from build123d import *

# Parameters (mm, degrees)
SKETCH1_W           = 66.4
SKETCH1_H           = 66.4
BOSS_EXTRUDE1_DEPTH = 59
SKETCH2_R           = 19.075
SKETCH2_R_2         = 2.75
CUT_EXTRUDE1_DEPTH  = 111.900495941
SKETCH3_W           = 57.4
SKETCH3_H           = 54.5
CUT_EXTRUDE2_DEPTH  = 61.9
CUT_EXTRUDE3_DEPTH  = 111.900495941
SKETCH5_W           = 116.4
SKETCH5_H           = 59
BOSS_EXTRUDE2_DEPTH = 4.5
SKETCH6_R           = 2.2
CUT_EXTRUDE4_DEPTH  = 126.166169551


with BuildPart() as part:
    # Sketch1 → Boss-Extrude1 (new body)
    with BuildSketch(Plane.XY):
        with Locations((33.2, 33.2)):
            Rectangle(SKETCH1_W, SKETCH1_H)
    extrude(amount=BOSS_EXTRUDE1_DEPTH)

    # Sketch2 → Cut-Extrude1 (cut, through all)
    with BuildSketch(Plane.XY.offset(59)):
        with Locations((33.2, 33.2)):
            Circle(SKETCH2_R)
        with Locations((9.63, 56.77)):
            Circle(SKETCH2_R_2)
        with Locations((56.77, 56.77)):
            Circle(SKETCH2_R_2)
        with Locations((56.77, 9.63)):
            Circle(SKETCH2_R_2)
        with Locations((9.63, 9.63)):
            Circle(SKETCH2_R_2)
    extrude(amount=-CUT_EXTRUDE1_DEPTH, mode=Mode.SUBTRACT)

    # Sketch3 → Cut-Extrude2 (cut)
    with BuildSketch(Plane(origin=(0, 66.4, 0), x_dir=(1, 0, 0), z_dir=(0, 1, 0))):
        with Locations((33.2, -27.25)):
            Rectangle(SKETCH3_W, SKETCH3_H)
    extrude(amount=-CUT_EXTRUDE2_DEPTH, mode=Mode.SUBTRACT)

    # Sketch4 → Cut-Extrude3 (cut, through all)
    with BuildSketch(Plane(origin=(66.4, 0, 0), x_dir=(0, 0, -1), z_dir=(1, 0, 0))):
        Polygon((-54.5, 66.4), (0, 66.4), (0, 4.5), align=None)
    extrude(amount=-CUT_EXTRUDE3_DEPTH, mode=Mode.SUBTRACT)

    # Sketch5 → Boss-Extrude2 (add)
    with BuildSketch(Plane.XZ):
        with Locations((33.2, 29.5)):
            Rectangle(SKETCH5_W, SKETCH5_H)
    extrude(amount=-BOSS_EXTRUDE2_DEPTH)

    # Sketch6 → Cut-Extrude4 (cut, through all)
    with BuildSketch(Plane(origin=(0, 4.5, 0), x_dir=(1, 0, 0), z_dir=(0, 1, 0))):
        with Locations(Location((-16.8, -9.5, 0), (0, 0, 270))):
            Circle(SKETCH6_R)
        with Locations(Location((-16.8, -49.5, 0), (0, 0, 270))):
            Circle(SKETCH6_R)
        with Locations(Location((83.2, -49.5, 0), (0, 0, 270))):
            Circle(SKETCH6_R)
        with Locations(Location((83.2, -9.5, 0), (0, 0, 270))):
            Circle(SKETCH6_R)
    extrude(amount=-CUT_EXTRUDE4_DEPTH, mode=Mode.SUBTRACT)


solid = part.part
For this review, take the finished solid that the model builds, in its own axes (mm). A direction names the side the tool comes from. Round coordinates to 2 decimals unless told otherwise and drop trailing zeros. Write each loop counter-clockwise with the first axis right and the second up, starting at its lowest first coordinate (ties: lowest second). Pieces come first, ordered by that corner, then holes. Notation, with made-up numbers: M 36.5,59 L 59.5,59 A19 ccw 59.5,71 Z; hole C 34,79.5 d6. An arc over 180 degrees is marked long. Write item = value, one per line. Start each with the question number.
(1) For line 1 along Y through (x, z) = (56.77, 56.25); line 2 along X through (y, z) = (14.5, 28); line 3 along X through (y, z) = (12, 56), list the stretches that pass through material, from the lowest coordinate up.
(2) Clearance check with flat-ended pins moving along their axes: pin 1 Ø6 at (y, z) = (13, 18) entering from -X; pin 2 Ø5 at (y, z) = (58.5, 43) entering from +X; pin 3 Ø4 at (y, z) = (25.5, 35) entering from +X; pin 4 Ø12.5 at (x, z) = (80.5, 28) entering from +Y. State where each tip first meets the part, or that it passes through.
(3) We need section A-A (x = 33.2). Give the boundary of the cut face in (y, z) (3 decimals), then the cut area to 3 significant figures.
(4) We need section D-D (y = 9.63). Give the boundary of the cut face in (x, z).
(5) We need section C-C (y = 24.5). Give the boundary of the cut face in (x, z).
(6) The part is to be moulded in two halves that separate along Z. For faces 4 (the face through (32, 2, 0)), 5 (the face through (-18.139, 2.282, 47.754)), 6 (the face through (66.4, 28, 36)), say which applies: +Z half, -Z half, draft (parallel to the pull), parting line (faces both ways), or undercut.
(7) We need section B-B (z = 9.5). Give the boundary of the cut face in (x, y), then the cut area to 3 significant figures.
(8) For faces 1 (the face through (64.18, 35.02, 26.87)), 2 (the face through (4.5, 22, 40)), 3 (the face through (79, 4.5, 30)), list the 3-axis set-ups (+Z, -Z, +X, -X, +Y, -Y) from which the entire face can be reached by the end or side of a thin tool; tool diameter is ignored.
Results found:
q1.line_1 = 0 to 6.88, 12.38 to 54.02, 59.52 to 66.4
q1.line_2 = 0 to 4.5, 61.9 to 66.4
q1.line_3 = 0 to 8.24, 11.02 to 55.38, 58.16 to 66.4
q2.pin_1 = 0
q2.pin_2 = through
q2.pin_3 = 66.4
q2.pin_4 = 4.5
q3.outline = M 0,0 L 4.5,0 L 4.5,54.5 L 14.125,54.5 L 14.125,59 L 0,59 Z; M 52.275,54.5 L 66.4,54.5 L 66.4,59 L 52.275,59 Z
q3.area = 372 mm²
q4.outline = M 0,4.52 L 4.5,4.52 L 4.5,54.5 L 6.88,54.5 L 6.88,59 L 0,59 Z; M 12.38,54.5 L 54.02,54.5 L 54.02,59 L 12.38,59 Z; M 59.52,54.5 L 61.9,54.5 L 61.9,4.52 L 66.4,4.52 L 66.4,59 L 59.52,59 Z
q5.outline = M 0,17.61 L 4.5,17.61 L 4.5,54.5 L 16.22,54.5 L 16.22,59 L 0,59 Z; M 50.18,54.5 L 61.9,54.5 L 61.9,17.61 L 66.4,17.61 L 66.4,59 L 50.18,59 Z
q6.face_4 = -Z half
q6.face_5 = undercut
q6.face_6 = draft
q7.outline = M -25,0 L -19,0 L -19,4.5 L -25,4.5 Z; M -14.6,0 L 81,0 L 81,4.5 L 66.4,4.5 L 66.4,15.29 L 61.9,15.29 L 61.9,4.5 L 4.5,4.5 L 4.5,15.29 L 0,15.29 L 0,4.5 L -14.6,4.5 Z; M 85.4,0 L 91.4,0 L 91.4,4.5 L 85.4,4.5 Z
q7.area = 581 mm²
q8.face_1 = -Z, +X, -X, +Y
q8.face_2 = -Z, +Y
q8.face_3 = +Z, -Z, +X, +Y
